```python
from build123d import *

# Parameters (mm, degrees)
ESQUISSE1_W        = 5
ESQUISSE1_H        = 40
ESQUISSE1_R        = 1.75
ESQUISSE1_W_2      = 20
BOSS_EXTRU_1_DEPTH = 2
ESQUISSE1_3_W      = 5
ESQUISSE1_3_H      = 40
ESQUISSE1_3_R      = 1.75
BOSS_EXTRU_2_DEPTH = 1


with BuildPart() as part:
    # Esquisse1 → Boss.-Extru.1 (new body)
    with BuildSketch(Plane.XY):
        with Locations((-12.5, 0)):
            Rectangle(ESQUISSE1_W, ESQUISSE1_H)
        with Locations((-12.5, -15)):
            Circle(ESQUISSE1_R, mode=Mode.SUBTRACT)
        with Locations((-12.5, 15)):
            Circle(ESQUISSE1_R, mode=Mode.SUBTRACT)
        Rectangle(ESQUISSE1_W_2, ESQUISSE1_H)
        with Locations((-7.25, -4.75)):
            Circle(ESQUISSE1_R, mode=Mode.SUBTRACT)
        with Locations((7.25, -4.75)):
            Circle(ESQUISSE1_R, mode=Mode.SUBTRACT)
        with Locations((-7.25, 4.75)):
            Circle(ESQUISSE1_R, mode=Mode.SUBTRACT)
        with Locations((7.25, 4.75)):
            Circle(ESQUISSE1_R, mode=Mode.SUBTRACT)
        with Locations((12.5, 0)):
            Rectangle(ESQUISSE1_W, ESQUISSE1_H)
        with Locations((12.5, -15)):
            Circle(ESQUISSE1_R, mode=Mode.SUBTRACT)
        with Locations((12.5, 15)):
            Circle(ESQUISSE1_R, mode=Mode.SUBTRACT)
    extrude(amount=-BOSS_EXTRU_1_DEPTH)

    # Esquisse1_3 → Boss.-Extru.2 (add)
    with BuildSketch(Plane.XY):
        with Locations((-12.5, 0)):
            Rectangle(ESQUISSE1_3_W, ESQUISSE1_3_H)
        with Locations((-12.5, -15)):
            Circle(ESQUISSE1_3_R, mode=Mode.SUBTRACT)
        with Locations((-12.5, 15)):
            Circle(ESQUISSE1_3_R, mode=Mode.SUBTRACT)
        with Locations((12.5, 0)):
            Rectangle(ESQUISSE1_3_W, ESQUISSE1_3_H)
        with Locations((12.5, -15)):
            Circle(ESQUISSE1_3_R, mode=Mode.SUBTRACT)
        with Locations((12.5, 15)):
            Circle(ESQUISSE1_3_R, mode=Mode.SUBTRACT)
    extrude(amount=BOSS_EXTRU_2_DEPTH)


solid = part.part
```
For this review, take the finished solid that the model builds, in its own axes (mm). A direction names the side the tool comes from. Round coordinates to 2 decimals unless told otherwise and drop trailing zeros. Write each loop counter-clockwise with the first axis right and the second up, starting at its lowest first coordinate (ties: lowest second). Pieces come first, ordered by that corner, then holes. Notation, with made-up numbers: (-29, -32.75) - (-5, -32.75) arc R26 ccw to (-5, -3.75) - close; hole circle Ø2 at (43, -30). An arc over 180 degrees is marked (long way). Put each result on its own line as item: value.
Q1. Insertion check: pin 1 Ø4 at (x, y) = (7.25, -4.75) entering from +Z; pin 2 Ø4.5 at (x, y) = (-12.5, 15) entering from +Z. Each pin has a flat end and moves straight along its axis. Give the tip position at first contact, or say it passes through.
Solved:
pin 1: stops at z = 0
pin 2: stops at z = 1
Q2. Mouldability with a two-part tool opening along Y and no side actions: class faces 1 (the face through (-5.633, -5.42, -0.986)), 2 (the face through (8.867, -5.42, -0.986)), 3 (the face through (12, 0, 1)), 4 (the face through (0, 20, -1)) as released by +Y, released by -Y, zero draft, split by the parting line, or undercut.
Solved:
face 1: undercut
face 2: undercut
face 3: zero draft
face 4: released by +Y
Q3. We need section D-D (y = -4.75). Give the boundary of the cut face in (x, z).
Solved:
outline: (-15, -2) - (-9, -2) - (-9, 0) - (-10, 0) - (-10, 1) - (-15, 1) - close; (-5.5, -2) - (5.5, -2) - (5.5, 0) - (-5.5, 0) - close; (9, -2) - (15, -2) - (15, 1) - (10, 1) - (10, 0) - (9, 0) - close
Q4. We need section B-B (x = 7.25). Give the boundary of the cut face in (y, z), and give its area (3 significant figures).
Solved:
outline: (-20, -2) - (-6.5, -2) - (-6.5, 0) - (-20, 0) - close; (-3, -2) - (3, -2) - (3, 0) - (-3, 0) - close; (6.5, -2) - (20, -2) - (20, 0) - (6.5, 0) - close
area: 66.0 mm2
Q5. Machinability: for faces 5 (the face through (-6.44, 3.2, -0.99)), 6 (the face through (0, 0, 0)), which of the approach directions +Z, -Z, +X, -X, +Y, -Y give a long, thin tool a straight path to every point of the face, cutting with its end or side? Answer none if there is none.
Solved:
face 5: +Z, -Z
face 6: +Z, +Y, -Y
Q6. We need section A-A (y = -15). Give the boundary of the cut face in (x, z).
Solved:
outline: (-15, -2) - (-14.25, -2) - (-14.25, 1) - (-15, 1) - close; (-10.75, -2) - (10.75, -2) - (10.75, 1) - (10, 1) - (10, 0) - (-10, 0) - (-10, 1) - (-10.75, 1) - close; (14.25, -2) - (15, -2) - (15, 1) - (14.25, 1) - close
Q7. We need section C-C (z = -0.45). Count the separate pieces of the cut face and the enclosed holes in it, and give its area (3 significant figures).
Solved:
separate pieces: 1
enclosed holes: 8
area: 1,120 mm2
Q8. Wall thickness on probe 1 along Y at (x, z) = (-7.25, -0.6); probe 2 along Y at (x, z) = (-12.5, 0.45); probe 3 along X at (y, z) = (-4, -1.7): over which ranges is each line inside the solid? List them lowest first.
Solved:
probe 1: y = -20 to -6.5, -3 to 3, 6.5 to 20
probe 2: y = -20 to -16.75, -13.25 to 13.25, 16.75 to 20
probe 3: x = -15 to -8.83, -5.67 to 5.67, 8.83 to 15
